The model under review builds one solid part; all positions refer to its coordinate system, in mm. A direction names the side the tool comes from. Round coordinates to 2 decimals unless told otherwise and drop trailing zeros. Order: outer loops, then holes, each group sorted by start corner. A loop starts at its lowest first (then second) coordinate and runs counter-clockwise, first axis right, second up. Notation, with made-up numbers: (32.5, -38.75) -> (77.5, -38.75) arc R16 ccw to (77.5, -27.75) -> close; hole circle Ø3 at (-31.75, 66.25). An arc over 180 degrees is marked (long way). Use a Markdown table: item, result. Add a question column.
```python
from build123d import *

# Parameters (mm, degrees)
CUT_EXTRUDE_1_DEPTH = 4


with BuildPart() as part:
    # Sketch 1 → Revolve 1 (revolve)
    with BuildSketch(Plane.XY, mode=Mode.PRIVATE) as revolve_1_sk:
        Polygon((-5, 0), (-5, 2), (-0.5, 2), (-0.5, 1.3), (0, 1.3), (0, 2.067), (0.433, 2.5), (25, 2.5), (25, 4.25), (29.292893219, 4.25), (30, 3.542893219), (30, 0), align=None)
    revolve(revolve_1_sk.sketch.rotate(Axis((30, 0, 0), (-1, 0, 0)), 270), axis=Axis((30, 0, 0), (-1, 0, 0)))

    # Sketch 2 → Cut-Revolve 1 (revolve, cut)
    with BuildSketch(Plane.XY, mode=Mode.PRIVATE) as cut_revolve_1_sk:
        Polygon((24.845299462, 0), (26, 2), (30, 2), (30, 0), align=None)
    revolve(cut_revolve_1_sk.sketch.rotate(Axis((30, 0, 0), (-1, 0, 0)), 270), axis=Axis((30, 0, 0), (-1, 0, 0)), mode=Mode.SUBTRACT)

    # Sketch 3 → Cut-Extrude 1 (cut)
    with BuildSketch(Plane(origin=(30, 0, 0), x_dir=(0, 0, -1), z_dir=(1, 0, 0))):
        Polygon((-2, 1.154700538), (-2, -1.154700538), (0, -2.309401077), (2, -1.154700538), (2, 1.154700538), (0, 2.309401077), align=None)
    extrude(amount=-CUT_EXTRUDE_1_DEPTH, mode=Mode.SUBTRACT)


solid = part.part
```
Q1. Wall thickness on line 1 (Y direction, x = 14, z = 0); line 2 (X direction, y = 1, z = 3); line 3 (Z direction, x = 15.5, y = 1.5): over which ranges is each line inside the solid? List them lowest first. Write a range as [from, to].
Q2. Add section B-B (x = -1.5). Write out the cut boundary in (y, z).
Q3. Machinability: for faces 1 (the cylindrical face through (-3, -2, 0)), 2 (the flat face through (28.028, -1.724, 1.014)), 3 (the cylindrical face through (27.176, 4.214, -0.553)), which of the approach directions +Z, -Z, +X, -X, +Y, -Y give a long, thin tool a straight path to every point of the face, cutting with its end or side? Answer none if there is none.
Q4. Mouldability with a two-part tool opening along X and no side actions: class faces 4 (the flat face through (28.03, -1.74, -0.99)), 5 (the flat face through (25, -2, -2)), 6 (the cylindrical face through (-0.25, 0.39, 1.24)), 7 (the conical face through (25.046, -0.339, -0.075)) as pulls with the +X half, pulls with the -X half, needs draft (parallel to the pull), parting line crosses it, or undercut.
Q5. Add section A-A (x = 17). Write out the cut boundary in (y, z).
Q6. Insertion check: pin 1 (2 mm diameter, centred on x = 17, y = 1, fed in from -Z); pin 2 (1.2 mm diameter, centred on y = 0, z = 0, fed in from +X); pin 3 (3 mm diameter, centred on x = 26, z = 2, fed in from +Y). Each pin has a flat end and moves straight along its axis. Give the tip position at first contact, or say it passes through.
Report:
| question | item | result |
|---|---|---|
| 1 | line 1 | y = [-2.5, 2.5] |
| 1 | line 2 | x = [25, 30] |
| 1 | line 3 | z = [-2, 2] |
| 2 | outline | circle Ø4 at (0, 0) |
| 3 | face 1 | -X |
| 3 | face 2 | +X |
| 3 | face 3 | +X, -X |
| 4 | face 4 | needs draft |
| 4 | face 5 | pulls with the -X half |
| 4 | face 6 | undercut |
| 4 | face 7 | pulls with the +X half |
| 5 | outline | circle Ø5 at (0, 0) |
| 6 | pin 1 | stops at z = -2.5 |
| 6 | pin 2 | stops at x = 25.19 |
| 6 | pin 3 | stops at y = 4.22 |
